Read the model definition and answer for the solid it produces. Units are mm, in the model's axes. Coordinates: 2 decimals unless noted, no trailing zeros. Order: outer loops, then holes, each group sorted by start corner. A loop starts at its lowest first (then second) coordinate and runs counter-clockwise, first axis right, second up. Notation, with made-up numbers: (-31.75, 8) -> (3.25, 8) arc R25 ccw to (3.25, 46) -> close; hole circle Ø6 at (83.5, 28). An arc over 180 degrees is marked (long way). Use CSV: the item, a comma, the result in double quotes.
```python
from build123d import *

# Parameters (mm, degrees)
SKETCH1_R           = 4
SKETCH1_R_2         = 3
BOSS_EXTRUDE1_DEPTH = 1.25
CHAMFER1_SIZE       = 0.1


with BuildPart() as part:
    # Sketch1 → Boss-Extrude1 (new body, symmetric)
    with BuildSketch(Plane(origin=(0, 0, 0), x_dir=(1, 0, 0), z_dir=(0, 1, 0))):
        with BuildLine():
            Line((-29.631837738, -67.163637426), (14.031469945, -56.277152124))
            ThreePointArc((14.031469945, -56.277152124), (18.738560702, -52.973221742), (20.01308876, -47.36534892))
            Line((20.01308876, -47.36534892), (13.793825748, -4.528855104))
            ThreePointArc((13.793825748, -4.528855104), (13.529290218, -0.271510867), (13.964419925, 3.971792226))
            Line((13.964419925, 3.971792226), (21.92672411, 46.682103314))
            ThreePointArc((21.92672411, 46.682103314), (14.515313736, 58.217743577), (2.555771725, 51.511824185))
            Line((2.555771725, 51.511824185), (-12.402419972, 3.896149233))
            ThreePointArc((-12.402419972, 3.896149233), (-12.997382983, -0.260836353), (-12.236118289, -4.390604654))
            Line((-12.236118289, -4.390604654), (-0.66120456, -36.648579291))
            ThreePointArc((-0.66120456, -36.648579291), (-1.017383505, -41.503892695), (-4.857112397, -44.496786566))
            Line((-4.857112397, -44.496786566), (-33.502588067, -51.638905806))
            ThreePointArc((-33.502588067, -51.638905806), (-39.329578713, -61.336646781), (-29.631837738, -67.163637426))
        make_face()
        Circle(SKETCH1_R, mode=Mode.SUBTRACT)
        with Locations((12.09609478, 48.514786314)):
            Circle(SKETCH1_R, mode=Mode.SUBTRACT)
        with Locations((7.257656868, 29.108871788)):
            Circle(SKETCH1_R_2, mode=Mode.SUBTRACT)
        with Locations((12.09609478, -48.514786314)):
            Circle(SKETCH1_R_2, mode=Mode.SUBTRACT)
        with Locations((-31.567212902, -59.401271616)):
            Circle(SKETCH1_R_2, mode=Mode.SUBTRACT)
    extrude(amount=BOSS_EXTRUDE1_DEPTH, both=True)

    # Chamfer1
    chamfer1_edges = [part.edges().sort_by_distance(p)[0] for p in [
        (-39.329578713, 1.25, 61.336646781),
        (-6.448661425, -1.25, 20.519591973),
        (-12.997382983, -1.25, 0.260836353),
        (-4.923324123, -1.25, -27.703986709),
        (14.515313736, -1.25, -58.217743577),
        (17.945572018, -1.25, -25.32694777),
        (13.529290218, -1.25, 0.271510867),
        (-7.800183896, 1.25, 61.720394775),
        (16.903457254, -1.25, 25.947102012),
        (18.738560702, -1.25, 52.973221742),
        (-7.800183896, -1.25, 61.720394775),
        (-39.329578713, -1.25, 61.336646781),
        (-19.179850232, -1.25, 48.067846186),
        (-1.017383505, -1.25, 41.503892695),
        (18.738560702, 1.25, 52.973221742),
        (16.903457254, 1.25, 25.947102012),
        (13.529290218, 1.25, 0.271510867),
        (17.945572018, 1.25, -25.32694777),
        (14.515313736, 1.25, -58.217743577),
        (-4, -1.25, 0),
        (-4, 1.25, 0),
        (-4.923324123, 1.25, -27.703986709),
        (8.09609478, -1.25, -48.514786314),
        (8.09609478, 1.25, -48.514786314),
        (-12.997382983, 1.25, 0.260836353),
        (-6.448661425, 1.25, 20.519591973),
        (4.257656868, -1.25, -29.108871788),
        (4.257656868, 1.25, -29.108871788),
        (-1.017383505, 1.25, 41.503892695),
        (9.09609478, -1.25, 48.514786314),
        (9.09609478, 1.25, 48.514786314),
        (-34.567212902, -1.25, 59.401271616),
        (-34.567212902, 1.25, 59.401271616),
        (-19.179850232, 1.25, 48.067846186),
    ]]
    chamfer(chamfer1_edges, length=CHAMFER1_SIZE)


solid = part.part
```
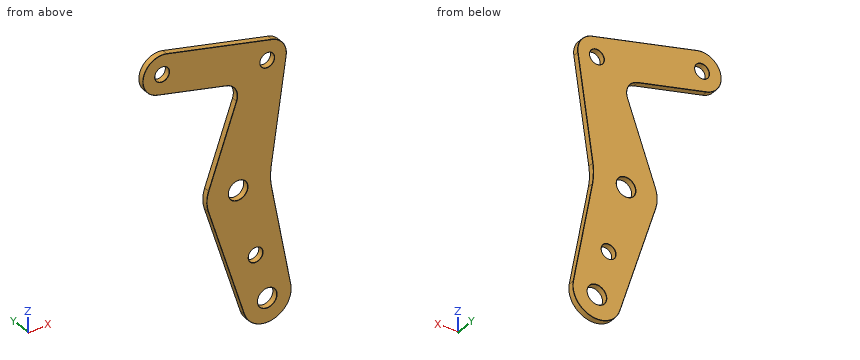
Item 1: Find section B-B, the plane z = 11.5. Give the vertices of the cut face in (x, y), then the cut area to 3 significant figures.
Return value:
outline,"(-9.69, -1.15) -> (-9.58, -1.25) -> (14.7, -1.25) -> (14.81, -1.15) -> (14.81, 1.15) -> (14.7, 1.25) -> (-9.58, 1.25) -> (-9.69, 1.15) -> close"
area,"61.2 mm^2"
Item 2: Find section A-A, the plane y = -0.2. Give the vertices of the cut face in (x, z), then the cut area to 3 significant figures.
Return value:
outline,"(-33.5, 51.64) -> (-4.86, 44.5) arc R6 cw to (-0.66, 36.65) -> (-12.24, 4.39) arc R13 ccw to (-12.4, -3.9) -> (2.56, -51.51) arc R10 ccw to (21.93, -46.68) -> (13.96, -3.97) arc R26 cw to (13.79, 4.53) -> (20.01, 47.37) arc R8 ccw to (14.03, 56.28) -> (-29.63, 67.16) arc R8 ccw to start; hole circle Ø6 at (-31.57, 59.4); hole circle Ø8 at (0, 0); hole circle Ø6 at (7.26, -29.11); hole circle Ø8 at (12.1, -48.51); hole circle Ø6 at (12.1, 48.51)"
area,"2,990 mm^2"
Item 3: Straight lines are drawn through the part: line 1 along X through (y, z) = (0.65, 0); line 2 along Z through (x, y) = (8.5, 0); line 3 along X through (y, z) = (0.5, -3). For each, find the intervals that lie inside material, in ascending order.
Return value:
line 1,"x = -13 to -4, 4 to 13.54"
line 2,"z = -57.85 to -50.27, -46.76 to -31.84, -26.38 to 57.66"
line 3,"x = -12.65 to -2.65, 2.65 to 13.8"
Item 4: Find section C-C, the plane x = -24. Give the vertices of the cut face in (y, z).
Return value:
outline,"(-1.25, 49.37) -> (-1.15, 49.27) -> (1.15, 49.27) -> (1.25, 49.37) -> (1.25, 65.66) -> (1.15, 65.76) -> (-1.15, 65.76) -> (-1.25, 65.66) -> close"
